Could you check a few things on this model? Use its own coordinates, in mm. Round coordinates to 2 decimals unless told otherwise and drop trailing zeros. Order: outer loops, then holes, each group sorted by start corner. A loop starts at its lowest first (then second) coordinate and runs counter-clockwise, first axis right, second up.
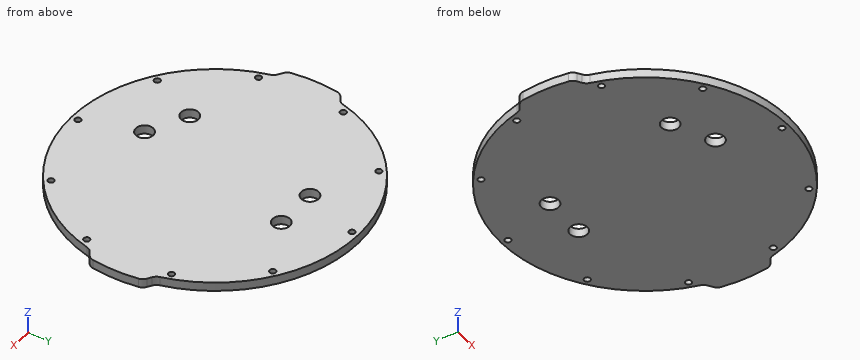
```python
from build123d import *

# Parameters (mm, degrees)
SKETCH1_R           = 1.75
SKETCH1_R_2         = 5
BOSS_EXTRUDE1_DEPTH = 2.54
FILLET1_R           = 5.08


with BuildPart() as part:
    # Sketch1 → Boss-Extrude1 (new, symmetric)
    with BuildSketch(Plane.XY):
        with BuildLine():
            Line((-86.162592811, 15.24), (-80.321852568, 19.05))
            ThreePointArc((-80.321852568, 19.05), (0, 82.55), (80.321852568, 19.05))
            Line((80.321852568, 19.05), (86.162592811, 15.24))
            ThreePointArc((86.162592811, 15.24), (87.5, 0), (86.162592811, -15.24))
            Line((86.162592811, -15.24), (80.321852568, -19.05))
            ThreePointArc((80.321852568, -19.05), (0, -82.55), (-80.321852568, -19.05))
            Line((-80.321852568, -19.05), (-86.162592811, -15.24))
            ThreePointArc((-86.162592811, -15.24), (-87.5, 0), (-86.162592811, 15.24))
        make_face()
        with Locations((0, 78.74)):
            Circle(SKETCH1_R, mode=Mode.SUBTRACT)
        with Locations((46.282210766, 63.701998137)):
            Circle(SKETCH1_R, mode=Mode.SUBTRACT)
        with Locations((74.886190093, 24.331998137)):
            Circle(SKETCH1_R, mode=Mode.SUBTRACT)
        with Locations((74.886190093, -24.331998137)):
            Circle(SKETCH1_R, mode=Mode.SUBTRACT)
        with Locations((46.282210766, -63.701998137)):
            Circle(SKETCH1_R, mode=Mode.SUBTRACT)
        with Locations((0, -78.74)):
            Circle(SKETCH1_R, mode=Mode.SUBTRACT)
        with Locations((-46.282210766, -63.701998137)):
            Circle(SKETCH1_R, mode=Mode.SUBTRACT)
        with Locations((-74.886190093, -24.331998137)):
            Circle(SKETCH1_R, mode=Mode.SUBTRACT)
        with Locations((-74.886190093, 24.331998137)):
            Circle(SKETCH1_R, mode=Mode.SUBTRACT)
        with Locations((-46.282210766, 63.701998137)):
            Circle(SKETCH1_R, mode=Mode.SUBTRACT)
        with Locations((-32.134671235, -35.656176248)):
            Circle(SKETCH1_R_2, mode=Mode.SUBTRACT)
        with Locations((-9.845967479, -46.979324435)):
            Circle(SKETCH1_R_2, mode=Mode.SUBTRACT)
        with Locations((-12.5, 46.343823752)):
            Circle(SKETCH1_R_2, mode=Mode.SUBTRACT)
        with Locations((12.5, 46.343823752)):
            Circle(SKETCH1_R_2, mode=Mode.SUBTRACT)
    extrude(amount=BOSS_EXTRUDE1_DEPTH, both=True)

    # Fillet1
    fillet1_edges = [part.edges().sort_by_distance(p)[0] for p in [
        (-86.162592811, 15.24, 0),
        (-80.321852568, 19.05, 0),
        (80.321852568, 19.05, 0),
        (86.162592811, 15.24, 0),
        (86.162592811, -15.24, 0),
        (80.321852568, -19.05, 0),
        (-80.321852568, -19.05, 0),
        (-86.162592811, -15.24, 0),
    ]]
    fillet(fillet1_edges, radius=FILLET1_R)


solid = part.part
```
Q1. Imagine slicing it at D-D, the plane x = 40.5. Please give me the cut outline in (y, z).
Q2. For P1, Ø16, axis at x = -9.85, y = -46.98, coming from the +Z side; P2, Ø1, axis at y = 51.5, z = 1, coming from the -X side; P3, Ø1, axis at x = -35, z = 0.5, coming from the -Y side (3 decimals); P4, Ø1, axis at y = 3.5, z = -0.5, coming from the -X side, each with a flat end and sliding along its axis, tell me the tip position at first contact or that it passes through.
Q3. Imagine slicing it at A-A, the plane y = -38.5. Please give me the cut outline in (x, z).
Q4. I need wall thicknesses on L1, parallel to Y at x = 47.5, z = 2.15; L2, parallel to Y at x = -45, z = 1.5; L3, parallel to X at y = -63, z = 0.9. Which ranges of each line are inside material? Lowest first, please.
Q5. Imagine slicing it at C-C, the plane z = 1.1. State how many separate pieces and enclosed holes the cut face has, then the cut area to 3 significant figures.
Q6. Imagine slicing it at B-B, the plane x = 15. Please give me the cut outline in (y, z), then the cut area to 3 significant figures.
Filled in:
1. outline: (-71.93, -2.54) - (71.93, -2.54) - (71.93, 2.54) - (-71.93, 2.54) - close
2. P1: stops at z = 2.54
2. P2: stops at x = -64.91
2. P3: stops at y = -74.995
2. P4: stops at x = -87.45
3. outline: (-73.02, -2.54) - (-36.25, -2.54) - (-36.25, 2.54) - (-73.02, 2.54) - close; (-28.02, -2.54) - (73.02, -2.54) - (73.02, 2.54) - (-28.02, 2.54) - close
4. L1: y = -67.51 to -64.96, -62.45 to 62.45, 64.96 to 67.51
4. L2: y = -69.21 to -64.89, -62.51 to 62.51, 64.89 to 69.21
4. L3: x = -53.34 to -47.89, -44.68 to 44.68, 47.89 to 53.34
5. separate pieces: 1
5. enclosed holes: 14
5. area: 21,300 mm2
6. outline: (-81.18, -2.54) - (42.01, -2.54) - (42.01, 2.54) - (-81.18, 2.54) - close; (50.67, -2.54) - (81.18, -2.54) - (81.18, 2.54) - (50.67, 2.54) - close
6. area: 781 mm2
